Read the model definition and answer for the solid it produces. Units are mm, in the model's axes. Face numbers are marked on the shaded views. Give positions to 0.01 mm unless a question says otherwise; leave off trailing zeros. Write each loop counter-clockwise with the first axis right and the second up, starting at its lowest first coordinate (ties: lowest second). Pieces come first, ordered by that corner, then holes. Notation, with made-up numbers: (39, -9) -> (77, -9) arc R11 cw to (77, 3) -> close; hole circle Ø3 at (89.25, -3). An arc over 180 degrees is marked (long way). Use a Markdown table: item, result.
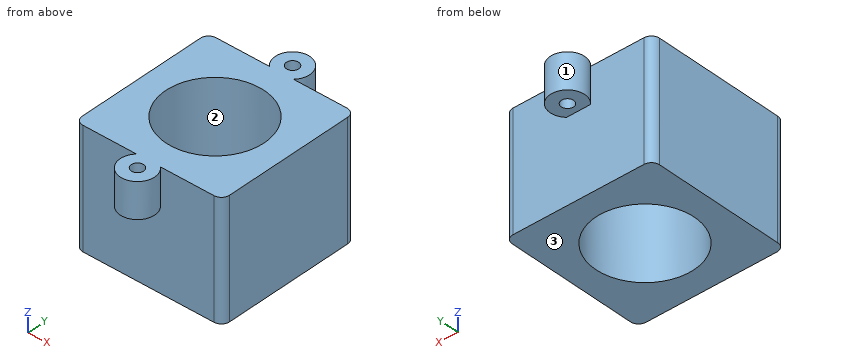
Autodesk Inventor part; units mm, degrees
ref_plane "YZ Plane" through (0, 0, 0) normal (1, 0, 0) x (0, 1, 0)
ref_plane "XZ Plane" through (0, 0, 0) normal (0, 1, 0) x (-1, 0, 0)
ref_plane "XY Plane" through (0, 0, 0) normal (0, 0, 1) x (1, 0, 0)
sketch "Skizze1" plane through (0, 0, 0) normal (0, 0, 1) x (1, 0, 0)
  line L0 (9, -9) -> (-9, -9)
  line L1 (-9, -9) -> (-9, 9)
  line L2 (-9, 9) -> (9, 9)
  line L3 (9, 9) -> (9, -9)
  line L4 (9, -9) -> (-9, 9) construction
  line L5 (-9, -9) -> (9, 9) construction
  circle A0 centre (0, 0) radius 6
  dimension "d0" = 18
  dimension "d1" = 18
  dimension "d2" = 12
extrude "Extrusion1" add sketch "Skizze1" along normal blind 10
fillet "Rundung1" radius 1 4 edges at (9, 9, 5) (-9, 9, 5) (9, -9, 5) (-9, -9, 5)
sketch "Skizze2" plane through (0, 0, 10) normal (0, 0, 1) x (1, 0, 0)
  arc A0 (-9, -8) -> (-8, -9) centre (-8, -8) ccw
  line L0 (-8, -9) -> (8, -9)
  arc A1 (8, -9) -> (9, -8) centre (8, -8) ccw
  line L1 (9, -8) -> (9, 8)
  arc A2 (9, 8) -> (8, 9) centre (8, 8) ccw
  line L2 (8, 9) -> (-8, 9)
  arc A3 (-8, 9) -> (-9, 8) centre (-8, 8) ccw
  line L3 (-9, 8) -> (-9, -8)
  circle A4 centre (0, 0) radius 6
  circle A5 centre (0, 10.5) radius 0.75
  circle A6 centre (0, -10.5) radius 0.75
  circle A7 centre (0, 10.5) radius 2.1
  circle A8 centre (0, -10.5) radius 2.1
  point P0 (-1.4697, -9)
  point P1 (1.4697, -9)
  point P2 (1.4697, 9)
  point P3 (-1.4697, 9)
  dimension "d6" = 1.5
  dimension "d7" = 1.5
  dimension "d8" = 10.5
  dimension "d9" = 10.5
  dimension "d10" = 4.2
  dimension "d11" = 4.2
extrude "Extrusion2" add sketch "Skizze2" along normal blind 4.3
properties part number "00_CCTV_M12_VCM_large"
Item 1: A cutting plane is placed at D-D (x = 3). Give the vertices of the cut face in (y, z), then the cut area to 3 significant figures.
Return value:
| item | result |
|---|---|
| outline | (-9, 0) -> (-5.2, 0) -> (-5.2, 14.3) -> (-9, 14.3) -> close; (5.2, 0) -> (9, 0) -> (9, 14.3) -> (5.2, 14.3) -> close |
| area | 109 mm^2 |
Item 2: A cutting plane is placed at B-B (z = 8.75). Give the vertices of the cut face in (x, y).
Return value:
| item | result |
|---|---|
| outline | (-9, -8) arc R1 ccw to (-8, -9) -> (8, -9) arc R1 ccw to (9, -8) -> (9, 8) arc R1 ccw to (8, 9) -> (-8, 9) arc R1 ccw to (-9, 8) -> close; hole circle Ø12 at (0, 0) |
Item 3: A cutting plane is placed at A-A (y = 10.5). Give the vertices of the cut face in (x, z), then the cut area to 3 significant figures.
Return value:
| item | result |
|---|---|
| outline | (-2.1, 10) -> (-0.75, 10) -> (-0.75, 14.3) -> (-2.1, 14.3) -> close; (0.75, 10) -> (2.1, 10) -> (2.1, 14.3) -> (0.75, 14.3) -> close |
| area | 11.6 mm^2 |
Item 4: Straight lines are drawn through the part: line 1 along Y through (x, z) = (0, 12.3); line 2 along X through (y, z) = (-1.5, 7.25); line 3 along Y through (x, z) = (1, 13.75). For each, find the intervals that lie inside material, in ascending order. Write a range as [from, to].
Return value:
| item | result |
|---|---|
| line 1 | [-12.6, -11.25], [-9.75, -6], [6, 9.75], [11.25, 12.6] |
| line 2 | [-9, -5.81], [5.81, 9] |
| line 3 | [-12.35, -5.92], [5.92, 12.35] |
Item 5: For a pull along Y with two mould halves and no side action, classify the marked faces 1, 2 and 3 as +Y half, -Y half, draft (parallel to the pull), parting line (faces both ways), or undercut.
Return value:
| item | result |
|---|---|
| face 1 | undercut |
| face 2 | undercut |
| face 3 | draft |
Item 6: A cutting plane is placed at C-C (x = 0). Give the vertices of the cut face in (y, z), then the cut area to 3 significant figures.
Return value:
| item | result |
|---|---|
| outline | (-12.6, 10) -> (-11.25, 10) -> (-11.25, 14.3) -> (-12.6, 14.3) -> close; (-9.75, 10) -> (-9, 10) -> (-9, 0) -> (-6, 0) -> (-6, 14.3) -> (-9.75, 14.3) -> close; (6, 0) -> (9, 0) -> (9, 10) -> (9.75, 10) -> (9.75, 14.3) -> (6, 14.3) -> close; (11.25, 10) -> (12.6, 10) -> (12.6, 14.3) -> (11.25, 14.3) -> close |
| area | 104 mm^2 |
Item 7: Each of these flat-tipped pins is pushed along its axis until it touches: P1, Ø1.4, axis at x = 0, y = -10.5, coming from the +Z side; P2, Ø2, axis at x = -0.5, z = 8, coming from the +Y side; P3, Ø5, axis at x = -6, z = 7.5, coming from the -Y side. Where does it stop, or does it pass through?
Return value:
| item | result |
|---|---|
| P1 | through |
| P2 | y = 9 |
| P3 | y = -9 |
